The model under review builds one solid part; all positions refer to its coordinate system, in mm. A direction names the side the tool comes from. Give positions to 0.01 mm unless a question says otherwise; leave off trailing zeros. Order: outer loops, then holes, each group sorted by start corner. A loop starts at its lowest first (then second) coordinate and runs counter-clockwise, first axis right, second up.
Autodesk Inventor part; units mm, degrees
ref_plane "YZ Plane" through (0, 0, 0) normal (1, 0, 0) x (0, 1, 0)
ref_plane "XZ Plane" through (0, 0, 0) normal (0, 1, 0) x (-1, 0, 0)
ref_plane "XY Plane" through (0, 0, 0) normal (0, 0, 1) x (1, 0, 0)
sketch "Sketch1" plane through (0, 0, 0) normal (0, 0, 1) x (1, 0, 0)
  circle A0 centre (0, 0) radius 28.3972
  dimension "d0" = 56.7944
extrude "Extrusion1" add sketch "Sketch1" along normal blind 5.9944
sketch "Sketch2" plane through (0, 0, 5.9944) normal (0, 0, 1) x (1, 0, 0)
  circle A0 centre (0, 0) radius 11.9888
  dimension "d3" = 23.9776
extrude "Extrusion2" add sketch "Sketch2" along normal blind 1.905
sketch "Sketch3" plane through (0, 0, 7.8994) normal (0, 0, 1) x (1, 0, 0)
  circle A0 centre (0, 0) radius 3.175
  dimension "d6" = 6.35
extrude "Extrusion3" cut sketch "Sketch3" against normal blind 25.4
sketch "Sketch4" plane through (0, 0, 5.9944) normal (0, 0, 1) x (1, 0, 0)
  circle A0 centre (0, 0) radius 28.3972
  circle A1 centre (0, 0) radius 11.9888
  circle A2 centre (0, 0) radius 28.3972
  circle A3 centre (0, 0) radius 28.3972
  point P0 (0.0446, 23.749)
hole "Hole1" at (0.0446, 23.749, 5.9944) direction (0, 0, -1) diameter 4.9784 depth 19.05 tip angle 118
pattern_circular "Circular Pattern1" count 6 over 360 about axis through (0, 0, 7.8994) along (0, 0, -1) of "Hole1"
properties part number "nexus adapter plate final"
Item 1: Take a section at B-B (z = 3.5). Give the boundary of the cut face in (x, y) (3 decimals), and give its area (3 significant figures).
Values found:
outline: circle Ø56.794 at (0, 0); hole circle Ø4.978 at (-20.59, -11.836); hole circle Ø4.978 at (-20.545, 11.913); hole circle Ø6.35 at (0, 0); hole circle Ø4.978 at (-0.045, -23.749); hole circle Ø4.978 at (0.045, 23.749); hole circle Ø4.978 at (20.545, -11.913); hole circle Ø4.978 at (20.59, 11.836)
area: 2,380 mm2
Item 2: Take a section at C-C (x = -6). Give the boundary of the cut face in (y, z), and give its area (3 significant figures).
Values found:
outline: (-27.76, 0) - (27.76, 0) - (27.76, 5.99) - (10.38, 5.99) - (10.38, 7.9) - (-10.38, 7.9) - (-10.38, 5.99) - (-27.76, 5.99) - close
area: 372 mm2
Item 3: Clearance check with flat-ended pins moving along their axes: pin 1 Ø6.5 at (x, y) = (-0.04, -23.75) entering from +Z; pin 2 Ø2 at (x, z) = (-9.5, 5.5) entering from -Y; pin 3 Ø5 at (x, y) = (-21, -18) entering from -Z; pin 4 Ø5 at (x, y) = (0, 0) entering from +Z. State where each tip first meets the part, or that it passes through.
Values found:
pin 1: stops at z = 5.99
pin 2: stops at y = -27.1
pin 3: stops at z = 0
pin 4: passes through
Item 4: For faces 5 (the cylindrical face through (-0.69, -3.1, 4)), 6 (the cylindrical face through (11.435, -3.601, 6.934)), list the 3-axis set-ups (+Z, -Z, +X, -X, +Y, -Y) from which the entire face can be reached by the end or side of a thin tool; tool diameter is ignored.
Values found:
face 5: +Z, -Z
face 6: +Z
Item 5: For line 1 (Y direction, x = 20.5, z = 5.5); line 2 (Y direction, x = -21.5, z = 4.5); line 3 (Z direction, x = -21, y = 16), list the stretches that pass through material, from the lowest coordinate up.
Values found:
line 1: y = -19.65 to -14.4, -9.42 to 9.35, 14.32 to 19.65
line 2: y = -18.55 to -14.15, -9.52 to 9.61, 14.21 to 18.55
line 3: z = 0 to 5.99
Item 6: Take a section at A-A (y = 0). Give the boundary of the cut face in (x, z) (3 decimals), and give its area (3 significant figures).
Values found:
outline: (-28.397, 0) - (-3.175, 0) - (-3.175, 7.899) - (-11.989, 7.899) - (-11.989, 5.994) - (-28.397, 5.994) - close; (3.175, 0) - (28.397, 0) - (28.397, 5.994) - (11.989, 5.994) - (11.989, 7.899) - (3.175, 7.899) - close
area: 336 mm2
Item 7: Draft analysis for pull direction X (two halves, no side actions). For faces 1 (the flat face through (2.5, -2.5, 7.899)), 2 (the cylindrical face through (0.065, -26.236, 2.955)), 3 (the cylindrical face through (-22.535, 17.279, 2.955)), 4 (the cylindrical face through (18.38, 12.98, 2.96)), state which applies: released by +X, released by -X, zero draft, split by the parting line, or undercut.
Values found:
face 1: zero draft
face 2: undercut
face 3: split by the parting line
face 4: undercut
Item 8: Take a section at D-D (y = 15.5). Give the boundary of the cut face in (x, z).
Values found:
outline: (-23.79, 0) - (23.79, 0) - (23.79, 5.99) - (-23.79, 5.99) - close
